Geometry check sheet. Reference: the model listing, model coordinates, mm. A direction names the side the tool comes from. Give positions to 0.01 mm unless a question says otherwise; leave off trailing zeros. Loops run counter-clockwise (first coordinate to the right, second up) from the corner with the lowest first, then second, coordinate; pieces in that order, holes last. Notation, with made-up numbers: (85.5, 57) - (116.5, 57) arc R15 cw to (116.5, 84) - close; hole circle Ø8 at (88, 22). An arc over 180 degrees is marked (long way). Use a Markdown table: item, result. Add a question column.
1. Cross-section at A-A on x = -9.25. Enter the section's corners in (y, z), and give its area (3 significant figures).
2. Material ranges on L1, parallel to Y at x = -12.7, z = -2.8; L2, parallel to X at y = 2.5, z = -6.25; L3, parallel to Z at x = -15.75, y = 4.5, recorded low to high.
3. Cross-section at D-D on y = 4.5. Enter the section's corners in (x, z).
4. Set-up check for faces 4 (the flat face through (-19.05, 4, -6)), 5 (the cylindrical face through (-11.274, 4.183, -1.972)): record each of +Z, -Z, +X, -X, +Y, -Y from which the full face is reachable in a straight line by a thin tool's end or side.
5. Draft check along X on faces 1 (the flat face through (-12.9, 6.4, -12.7)), 2 (the flat face through (0, 4, -6)), 3 (the flat face through (-11, 2, -3.81)). Enter one of: pulls with the +X half, pulls with the -X half, needs draft (parallel to the pull), parting line crosses it, or undercut.
6. Cross-section at B-B on z = -4.25. Enter the section's corners in (x, y).
7. Cross-section at C-C on x = -12.7. Enter the section's corners in (y, z).
Autodesk Inventor part; units mm, degrees
ref_plane "YZ Plane" through (0, 0, 0) normal (1, 0, 0) x (0, 1, 0)
ref_plane "XZ Plane" through (0, 0, 0) normal (0, 1, 0) x (-1, 0, 0)
ref_plane "XY Plane" through (0, 0, 0) normal (0, 0, 1) x (1, 0, 0)
sketch "Sketch1" plane through (0, 0, 0) normal (0, 1, 0) x (-1, 0, 0)
  line L0 (0, 0) -> (25.4, 0)
  line L1 (25.4, 0) -> (25.4, -12.7)
  line L2 (25.4, -12.7) -> (0, -12.7)
  line L3 (0, -12.7) -> (0, 0)
  line L4 (6.35, -3.81) -> (19.05, -3.81)
  line L5 (19.05, -3.81) -> (19.05, -8.5598)
  line L6 (19.05, -8.5598) -> (6.35, -8.5598)
  line L7 (6.35, -8.5598) -> (6.35, -3.81)
  dimension "d0" = 25.4
  dimension "d1" = 12.7
  dimension "d2" = 12.7
  dimension "d3" = 4.7498
  dimension "d5" = 6.35
  dimension "d6" = 3.81
extrude "Extrusion1" add sketch "Sketch1" along normal blind 9
sketch "Sketch2" plane through (-19.05, 0, -8.5598) normal (0, 0, 1) x (1, 0, 0)
  circle A0 centre (6.35, 4.5) radius 2.54
  line L0 (12.7, 0) -> (12.7, 9)
  point P0 (19.05, 0)
  dimension "d9" = 5.08
  dimension "d10" = 4.5
  dimension "d11" = 6.35
extrude "Extrusion2" add sketch "Sketch2" along normal blind 0.1905
sketch "Sketch3" plane through (-6.35, 0, -3.81) normal (0, 0, -1) x (-1, 0, 0)
  circle A0 centre (6.35, 4.5) radius 2.54
  line L0 (0, 0) -> (0, 9)
  point P0 (-6.35, 0)
  dimension "d14" = 5.08
  dimension "d15" = 4.5
  dimension "d16" = 6.35
extrude "Extrusion3" add sketch "Sketch3" along normal blind 0.1905
sketch "Sketch4" plane through (0, 0, -12.7) normal (0, 0, -1) x (-1, 0, 0)
  circle A0 centre (12.7, 4.5) radius 1.4605
  line L0 (0, 0) -> (0, 9)
  line L1 (25.4, 0) -> (0, 0)
  dimension "d19" = 2.921
  dimension "d20" = 12.7
  dimension "d21" = 4.5
hole "Hole1" at (-12.7, 4.5, -12.7) direction (0, 0, 1) diameter 2.921 end through all
properties part number "pulley enclosure test"
Values found:
| question | item | result |
|---|---|---|
| 1 | outline | (0, -12.7) - (9, -12.7) - (9, -8.56) - (0, -8.56) - close; (0, -3.81) - (9, -3.81) - (9, 0) - (0, 0) - close |
| 1 | area | 71.6 mm2 |
| 2 | L1 | y = 0 to 3.04, 5.96 to 9 |
| 2 | L2 | x = -25.4 to -19.05, -6.35 to 0 |
| 2 | L3 | z = -12.7 to -8.56, -3.81 to 0 |
| 3 | outline | (-25.4, -12.7) - (-14.16, -12.7) - (-14.16, -8.37) - (-15.24, -8.37) - (-15.24, -8.56) - (-19.05, -8.56) - (-19.05, -3.81) - (-15.24, -3.81) - (-15.24, -4) - (-14.16, -4) - (-14.16, 0) - (-25.4, 0) - close; (-11.24, -12.7) - (0, -12.7) - (0, 0) - (-11.24, 0) - (-11.24, -4) - (-10.16, -4) - (-10.16, -3.81) - (-6.35, -3.81) - (-6.35, -8.56) - (-10.16, -8.56) - (-10.16, -8.37) - (-11.24, -8.37) - close |
| 4 | face 4 | +Y, -Y |
| 4 | face 5 | +Z, -Z |
| 5 | face 1 | needs draft |
| 5 | face 2 | pulls with the +X half |
| 5 | face 3 | undercut |
| 6 | outline | (-25.4, 0) - (-19.05, 0) - (-19.05, 9) - (-25.4, 9) - close; (-6.35, 0) - (0, 0) - (0, 9) - (-6.35, 9) - close |
| 7 | outline | (0, -12.7) - (3.04, -12.7) - (3.04, -8.37) - (1.96, -8.37) - (1.96, -8.56) - (0, -8.56) - close; (0, -3.81) - (1.96, -3.81) - (1.96, -4) - (3.04, -4) - (3.04, 0) - (0, 0) - close; (5.96, -12.7) - (9, -12.7) - (9, -8.56) - (7.04, -8.56) - (7.04, -8.37) - (5.96, -8.37) - close; (5.96, -4) - (7.04, -4) - (7.04, -3.81) - (9, -3.81) - (9, 0) - (5.96, 0) - close |
